The model under review builds one solid part; all positions refer to its coordinate system, in mm. Face numbers are marked on the shaded views. A direction names the side the tool comes from. Coordinates: 2 decimals unless noted, no trailing zeros. Order: outer loops, then holes, each group sorted by start corner. A loop starts at its lowest first (then second) coordinate and runs counter-clockwise, first axis right, second up. Notation, with made-up numbers: M -30,62 L -5,62 A28 ccw -5,87 Z; hole C 29.5,-21 d2. An arc over 180 degrees is marked long. Answer as CSV lines item,"result". Start each with the question number.
Q1. For P1, Ø5, axis at x = -21, z = -12, coming from the -Y side; P2, Ø1.5, axis at x = -20, z = 15, coming from the -Y side; P3, Ø2.5, axis at x = -12, y = -0.5, coming from the +Z side; P4, Ø11.5, axis at x = 30, y = -5.5, coming from the -Z side, all flat-tipped, find the tip position at first contact; note any pin that passes through.
Q2. The part is to be moulded in two halves that separate along Y. For the marked faces 1, 2 and 3, say which applies: +Y half, -Y half, draft (parallel to the pull), parting line (faces both ways), or undercut.
Q3. Consider section A-A on y = 0. Write out the cut boundary in (x, z).
Q4. Machinability: for the marked faces 4, 5, 6 and 7, which of the approach directions +Z, -Z, +X, -X, +Y, -Y give a long, thin tool a straight path to every point of the face, cutting with its end or side? Answer none if there is none.
Q5. Consider section C-C on y = 10.5. Write out the cut boundary in (x, z), and give its area (3 significant figures).
Q6. Consider section B-B on x = 0.5. Write out the cut boundary in (y, z).
Q7. Consider section D-D on x = 10. Write out the cut boundary in (y, z), and give its area (3 significant figures).
Q8. Wall thickness on L1, parallel to Z at x = 19.5, y = 23; L2, parallel to X at y = 19, z = -6; L3, parallel to Y at x = -7, z = 0: over which ranges is each line inside the solid? List them lowest first. Write a range as [from, to].
from build123d import *

# Parameters (mm, degrees)
SKETCH1_W               = 16
SKETCH1_H               = 57
BOSS_EXTRUDE1_DEPTH     = 42
SKETCH3_R               = 8
BOSS_EXTRUDE4_DEPTH     = 14
SKETCH6_R               = 28.5
SKETCH6_R_2             = 15
BOSS_EXTRUDE5_DEPTH     = 36
CUT_EXTRUDE1_START      = -36
SKETCH8_R               = 15
CUT_EXTRUDE1_DEPTH      = 36
CUT_EXTRUDE3_DEPTH      = 104.325940596
CUT_EXTRUDE3_DEPTH_BACK = 104.325940596


with BuildPart() as part:
    # Sketch1 → Boss-Extrude1 (new, symmetric)
    with BuildSketch(Plane.XY):
        Rectangle(SKETCH1_W, SKETCH1_H)
    extrude(amount=BOSS_EXTRUDE1_DEPTH, both=True)

    # Sketch3 → Boss-Extrude4 (add)
    with BuildSketch(Plane(origin=(0, 0, -42), x_dir=(-1, 0, 0), z_dir=(0, 0, -1))):
        with BuildLine():
            Line((-33.275105345, 18.629891095), (-8, 28.5))
            Line((-8, 28.5), (-8, -28.5))
            Line((-8, -28.5), (-33.275105345, -18.629891095))
            ThreePointArc((-33.275105345, -18.629891095), (-46, 0), (-33.275105345, 18.629891095))
        make_face()
        with Locations((-26, 0)):
            Circle(SKETCH3_R, mode=Mode.SUBTRACT)
    boss_extrude4 = extrude(amount=-BOSS_EXTRUDE4_DEPTH)

    # Mirror6: Boss-Extrude4 across plane
    add(boss_extrude4.mirror(Plane.XY))

    # Sketch6 → Boss-Extrude5 (add)
    with BuildSketch(Plane.ZY.offset(8)):
        with Locations(Location((0, 0, 0), (0, 0, 270))):
            Circle(SKETCH6_R)
        with Locations(Location((0, 0, 0), (0, 0, 270))):
            Circle(SKETCH6_R_2, mode=Mode.SUBTRACT)
    extrude(amount=BOSS_EXTRUDE5_DEPTH)

    # Sketch8 → Cut-Extrude1 (cut)
    with BuildSketch(Plane.ZY.offset(8).offset(CUT_EXTRUDE1_START)):
        with Locations(Location((0, 0, 0), (0, 0, 270))):
            Circle(SKETCH8_R)
    extrude(amount=CUT_EXTRUDE1_DEPTH, mode=Mode.SUBTRACT)

    # Sketch9 → Cut-Extrude3 (cut, two sides: drawn at the far end of the back side and taken through both)
    with BuildSketch(Plane.ZY.offset(44).offset(-CUT_EXTRUDE3_DEPTH_BACK)):
        with BuildLine():
            ThreePointArc((-14.456832295, -4), (-14.863587797, -2.018355219), (-15, 0))
            Line((-15, 0), (-19, 0))
            Line((-19, 0), (-19, -4))
            Line((-19, -4), (-14.456832295, -4))
        make_face()
        with BuildLine():
            Line((-19, 0), (-15, 0))
            ThreePointArc((-15, 0), (-14.863587797, 2.018355219), (-14.456832295, 4))
            Line((-14.456832295, 4), (-19, 4))
            Line((-19, 4), (-19, 0))
        make_face()
        with BuildLine():
            ThreePointArc((-14.456832295, 4), (-14.863587797, 2.018355219), (-15, 0))
            ThreePointArc((-15, 0), (-14.863587797, -2.018355219), (-14.456832295, -4))
            Line((-14.456832295, -4), (-12.246493105, -4))
            Line((-12.246493105, -4), (-12.246493105, 4))
            Line((-12.246493105, 4), (-14.456832295, 4))
        make_face()
        with BuildLine():
            ThreePointArc((15, 0), (2.018355219, 14.863587797), (-14.456832295, 4))
            Line((-14.456832295, 4), (-12.246493105, 4))
            Line((-12.246493105, 4), (-12.246493105, -4))
            Line((-12.246493105, -4), (-14.456832295, -4))
            ThreePointArc((-14.456832295, -4), (2.018355219, -14.863587797), (15, 0))
        make_face()
    extrude(amount=CUT_EXTRUDE3_DEPTH + CUT_EXTRUDE3_DEPTH_BACK, mode=Mode.SUBTRACT)


solid = part.part
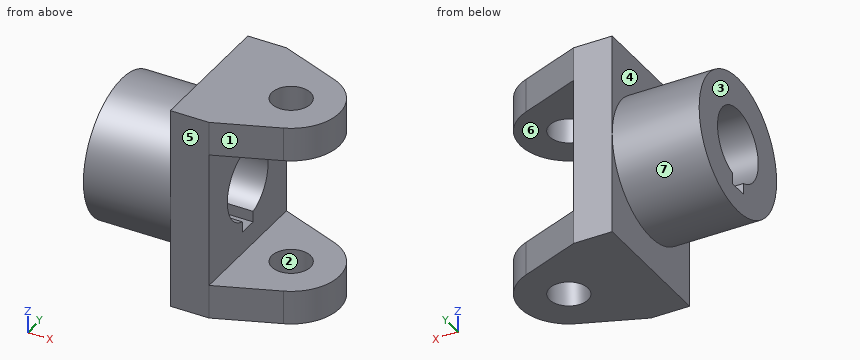
Evaluation:
1,P1,"stops at y = -26.87"
1,P2,"stops at y = -24.68"
1,P3,"stops at z = 28.5"
1,P4,"stops at z = -42"
2,face 1,"-Y half"
2,face 2,"undercut"
2,face 3,"draft"
3,outline,"M -44,-28.5 L -8,-28.5 L -8,-42 L 18,-42 L 18,-28 L 8,-28 L 8,-19 L -44,-19 Z; M -44,15 L 8,15 L 8,28 L 18,28 L 18,42 L -8,42 L -8,28.5 L -44,28.5 Z; M 34,-42 L 46,-42 L 46,-28 L 34,-28 Z; M 34,28 L 46,28 L 46,42 L 34,42 Z"
4,face 4,"+Z, -X"
4,face 5,"+Z, -Z, +X, -X, -Y"
4,face 6,"+X, +Y, -Y"
4,face 7,"-X"
5,outline,"M -44,-26.5 L -8,-26.5 L -8,-42 L 43.02,-42 L 43.02,-28 L 8,-28 L 8,-10.71 L -44,-10.71 Z; M -44,10.71 L 8,10.71 L 8,28 L 43.02,28 L 43.02,42 L -8,42 L -8,26.5 L -44,26.5 Z"
5,area,"3,120 mm²"
6,outline,"M -28.5,-42 L 28.5,-42 L 28.5,42 L -28.5,42 Z; hole M -4,-19 L 4,-19 L 4,-14.46 A15 ccw long -4,-14.46 Z"
7,outline,"M -27.72,-42 L 27.72,-42 L 27.72,-28 L -27.72,-28 Z; M -27.72,28 L 27.72,28 L 27.72,42 L -27.72,42 Z"
7,area,"1,550 mm²"
8,L1,"z = [-42, -28], [28, 42]"
8,L2,"x = [-44, 8]"
8,L3,"y = [-28.5, -15], [15, 28.5]"
